Here's how the part is built. I have some questions about the finished solid (model axes, mm). Face numbers are marked on the shaded views. A direction names the side the tool comes from. Coordinates: 2 decimals unless noted, no trailing zeros. Write each loop counter-clockwise with the first axis right and the second up, starting at its lowest first coordinate (ties: lowest second). Pieces come first, ordered by that corner, then holes.
Item 1: I'm going to push flat-ended pins straight in: P1, Ø13, axis at x = -1, z = 20.5, coming from the +Y side; P2, Ø2.5, axis at y = -2, z = 21, coming from the +X side; P3, Ø3.5, axis at x = -14.5, y = -1.5, coming from the +Z side. Where does each tip first touch, or does it pass through?
Item 2: I want a section at C-C (y = -1.25). Please give me the cut outline in (x, z).
Item 3: I want a section at A-A (z = 24.5). Please give me the cut outline in (x, y) (3 decimals).
Item 4: Please list where these lines run through material, in increasing order: line 1 (Z direction, x = 0, y = -2); line 2 (X direction, y = -0.5, z = -13); line 3 (Y direction, x = 10, z = -13) (1 decimal).
Item 5: For the marked faces 1, 2 and 3, which set-ups out of +Z, -Z, +X, -X, +Y, -Y let a thin tool reach every point of the face, with its end or its side?
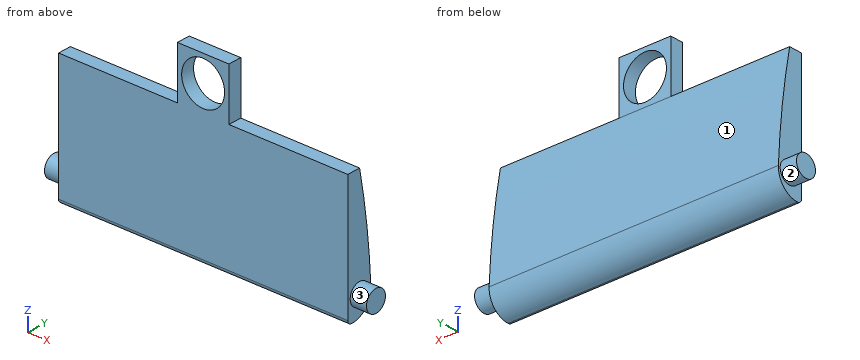
from build123d import *

# Parameters (mm, degrees)
F2_DEPTH = 3.125
F1_W     = 12
F1_H     = 12
F1_R     = 5
F3_DEPTH = 3.125
F4_R     = 2.5
F6_DEPTH = 3.81
F5_R     = 2.5
F7_DEPTH = 3.81
F8_DEPTH = 67.38
F9_R     = 5
F10_R    = 1


with BuildPart() as f2:
    # F1 (on Front) → F2 (new body, symmetric)
    with BuildSketch(Plane.XZ):
        Polygon((-6, 15), (-33.69, 15), (-33.69, -15), (33.69, -15), (33.69, 15), (6, 15), align=None)
    extrude(amount=F2_DEPTH, both=True)

    # F1 (on Front) → F3 (join, through all)
    with BuildSketch(Plane.XZ):
        with Locations((0, 21)):
            Rectangle(F1_W, F1_H)
        with Locations((0, 21)):
            Circle(F1_R, mode=Mode.SUBTRACT)
    extrude(amount=F3_DEPTH)

    # F4 (on face) → F6 (join)
    with BuildSketch(Plane.YZ.offset(33.69)):
        with Locations((0, -10)):
            Circle(F4_R)
    extrude(amount=F6_DEPTH)

    # F5 (on face) → F7 (join)
    with BuildSketch(Plane(origin=(-33.69, 0, 0), x_dir=(0, -1, 0), z_dir=(-1, 0, 0))):
        with Locations((0, -10)):
            Circle(F5_R)
    extrude(amount=F7_DEPTH)

    # F4 (on face) → F8 (cut, through all)
    with BuildSketch(Plane.YZ.offset(33.69)):
        with BuildLine():
            ThreePointArc((0, 15), (2.2291595567, 0.0694437038), (3.125, -15))
            Line((3.125, -15), (3.125, 15))
            Line((3.125, 15), (0, 15))
        make_face()
    extrude(amount=-F8_DEPTH, mode=Mode.SUBTRACT)

    # F9
    f9_edges = [f2.edges().sort_by_distance(p)[0] for p in [
        (0, 3.125, -15),
    ]]
    fillet(f9_edges, radius=F9_R)

    # F10
    f10_edges = [f2.edges().sort_by_distance(p)[0] for p in [
        (0, -3.125, -15),
    ]]
    fillet(f10_edges, radius=F10_R)


solid = f2.part
Answer:
1. P1: stops at y = 0.19
1. P2: stops at x = 6
1. P3: stops at z = 15
2. outline: (-37.5, -12.17) - (-33.69, -12.17) - (-33.69, -14.94) - (33.69, -14.94) - (33.69, -12.17) - (37.5, -12.17) - (37.5, -7.83) - (33.69, -7.83) - (33.69, 15) - (6, 15) - (6, 27) - (-6, 27) - (-6, 15) - (-33.69, 15) - (-33.69, -7.83) - (-37.5, -7.83) - close; hole circle Ø10 at (0, 21)
3. outline: (-6, -3.125) - (-3.571, -3.125) - (-3.571, 0) - (-6, 0) - close; (3.571, -3.125) - (6, -3.125) - (6, 0) - (3.571, 0) - close
4. line 1: z = -15 to 16, 26 to 27
4. line 2: x = -33.69 to 33.69
4. line 3: y = -3.1 to 2
5. face 1: +Z, +X, -X, +Y
5. face 2: -X
5. face 3: +X
